Can you work these out from the model? Positions are in its coordinate system, mm. A direction names the side the tool comes from. Round coordinates to 2 decimals unless told otherwise and drop trailing zeros. Loops run counter-clockwise (first coordinate to the right, second up) from the corner with the lowest first, then second, coordinate; pieces in that order, holes last.
from build123d import *

# Parameters (mm, degrees)
F0_W          = 410
F0_H          = 335
F0_W_2        = 385
F0_H_2        = 310
F1_DEPTH      = 22
F2_DEPTH      = 20
F4_DEPTH      = 480
F4_DEPTH_BACK = 70
F5_W          = 366
F5_H          = 239
F6_DEPTH      = 30
F7_R          = 29.99999
F9_W          = 550
F9_H          = 371
F10_DEPTH     = 2


# Not quite as in the source:
# - a fillet or chamfer is up to 0.001 mm smaller than in the source, because OpenCascade refuses the exact size


with BuildPart() as f1:
    # F0 (on Front) → F1 (new body)
    with BuildSketch(Plane.XZ):
        Rectangle(F0_W, F0_H)
        Rectangle(F0_W_2, F0_H_2, mode=Mode.SUBTRACT)
    extrude(amount=F1_DEPTH)

    # F0 (on Front) → F2 (join)
    with BuildSketch(Plane.XZ):
        Rectangle(F0_W_2, F0_H_2)
    extrude(amount=F2_DEPTH)

    # F5 (on face) → F6 (join)
    with BuildSketch(Plane(origin=(0, 0, 0), x_dir=(-1, 0, 0), z_dir=(0, 1, 0))):
        with Locations((0, 12)):
            Rectangle(F5_W, F5_H)
    extrude(amount=F6_DEPTH)

    # F7 (radius 30 in the source; OpenCascade refuses exactly that, so slightly less here)
    f7_edges = [f1.edges().sort_by_distance(p)[0] for p in [
        (-183, 30, 12),
        (0, 30, 131.5),
        (183, 30, 12),
        (0, 30, -107.5),
    ]]
    fillet(f7_edges, radius=F7_R)


with BuildPart() as f4:
    # F3 (on face) → F4 (new body, two sides)
    with BuildSketch(Plane.YZ.offset(205)) as f4_sk:
        Polygon((0, -167.5), (-22, -167.5), (-22, -185.5), (18, -185.5), (18, -146.5062479338), (0, -146.5062479338), align=None)
    extrude(amount=-F4_DEPTH)
    extrude(f4_sk.sketch, amount=F4_DEPTH_BACK)


with BuildPart() as f4b:
    # F3 (on face) → F4, piece 2 (new body, two sides)
    with BuildSketch(Plane.YZ.offset(205)) as f4_2_sk:
        Polygon((0, 146.5062479338), (18, 146.5062479338), (18, 185.5), (-22, 185.5), (-22, 167.5), (0, 167.5), align=None)
    extrude(amount=-F4_DEPTH)
    extrude(f4_2_sk.sketch, amount=F4_DEPTH_BACK)


with BuildPart() as f4_1:
    add(f4.part)

    # F8: union F4b, F1
    add(f4b.part)
    add(f1.part)

    # F9 (on face) → F10 (join)
    with BuildSketch(Plane.XZ.offset(22)):
        Rectangle(F9_W, F9_H)
    extrude(amount=F10_DEPTH)


solid = f4_1.part
(1) If we mould it in two halves opening along Y, with no side actions, what happens to faces 1 (the flat face through (240, -11, -167.5)), 2 (the flat face through (-275, -23, -1)), 3 (the cylindrical face through (174.445, 20.979, 13.673))? For each: released by +Y, released by -Y, zero draft, split by the parting line, or undercut.
Worked answers:
face 1: undercut
face 2: zero draft
face 3: released by +Y
(2) Will these pins go through, and if not, where does the flat tip stop? P1, Ø3, axis at y = 14, z = -64, coming from the -X side; P2, Ø11.5, axis at x = -9.5, z = -172.5, coming from the +Y side; P3, Ø4, axis at y = 2.5, z = 61, coming from the -X side; P4, Ø10, axis at y = 0.5, z = -146, coming from the -X side.
Worked answers:
P1: stops at x = -180.27
P2: stops at y = 18
P3: stops at x = -183
P4: stops at x = -275
(3) If we section it at B-B, the plane z = -119: List the corners of the cut face in (x, y) for me.
Worked answers:
outline: (-275, -24) - (275, -24) - (275, -22) - (205, -22) - (205, 0) - (-205, 0) - (-205, -22) - (-275, -22) - close; hole (-192.5, -22) - (192.5, -22) - (192.5, -20) - (-192.5, -20) - close
(4) If we section it at C-C, the plane y = -10: List the corners of the cut face in (x, z) for me, then the cut area to 3 significant figures.
Worked answers:
outline: (-275, -185.5) - (275, -185.5) - (275, -167.5) - (205, -167.5) - (205, 167.5) - (275, 167.5) - (275, 185.5) - (-275, 185.5) - (-275, 167.5) - (-205, 167.5) - (-205, -167.5) - (-275, -167.5) - close
area: 157,000 mm2
(5) If we section it at D-D, the plane x = 237: List the corners of the cut face in (y, z) for me, then the cut area to 3 significant figures.
Worked answers:
outline: (-24, -185.5) - (18, -185.5) - (18, -146.51) - (0, -146.51) - (0, -167.5) - (-22, -167.5) - (-22, 167.5) - (0, 167.5) - (0, 146.51) - (18, 146.51) - (18, 185.5) - (-24, 185.5) - close
area: 2,940 mm2
(6) If I drill on line 1 (Z direction, x = -157, y = 2); line 2 (Z direction, x = -26, y = 0.5); line 3 (Y direction, x = -93.5, z = -134), over which ranges is the centre line in solid material (lowest first)?
Worked answers:
line 1: z = -185.5 to -146.51, -107.43 to 131.43, 146.51 to 185.5
line 2: z = -185.5 to -146.51, -107.5 to 131.5, 146.51 to 185.5
line 3: y = -24 to -22, -20 to 0
(7) For faces 4 (the flat face through (-205, -11, -2)), 5 (the flat face through (-4, 18, 166)), 6 (the flat face through (-4, 9, 146.506)), which set-ups out of +Z, -Z, +X, -X, +Y, -Y let a thin tool reach every point of the face, with its end or its side?
Worked answers:
face 4: -X
face 5: +Z, +X, -X, +Y
face 6: +X, -X, +Y
